Input: part model. Units: mm. Frame: model coordinates. Face numbers are marked on the shaded views. A direction names the side the tool comes from. Round coordinates to 2 decimals unless told otherwise and drop trailing zeros. Write each loop counter-clockwise with the first axis right and the second up, starting at its lowest first coordinate (ties: lowest second). Pieces come first, ordered by that corner, then holes. Notation, with made-up numbers: M -30,-30 L -5,-30 A25 ccw -5,-3 Z; hole C -3,68.5 d1. An arc over 180 degrees is marked long. Answer as CSV lines item,"result". Start each with the question number.
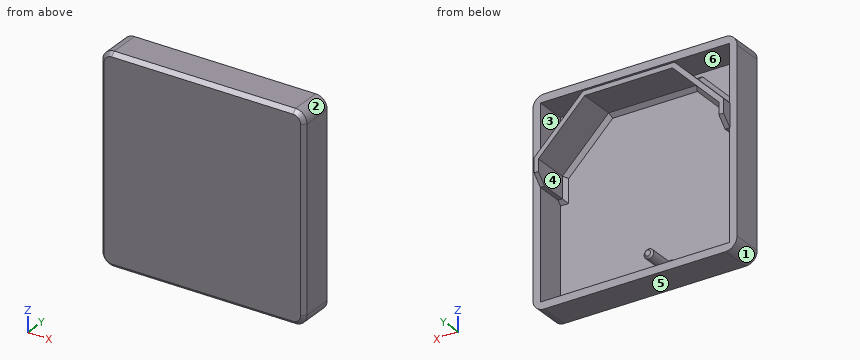
Autodesk Inventor part; units mm, degrees
ref_plane "YZ Plane" through (0, 0, 0) normal (1, 0, 0) x (0, 1, 0)
ref_plane "XZ Plane" through (0, 0, 0) normal (0, 1, 0) x (-1, 0, 0)
ref_plane "XY Plane" through (0, 0, 0) normal (0, 0, 1) x (1, 0, 0)
sketch "Náčrt1" plane through (0, 0, 0) normal (0, 1, 0) x (-1, 0, 0)
  line L0 (49.5, 49.5) -> (-49.5, 49.5)
  line L1 (-49.5, 49.5) -> (-49.5, -49.5)
  line L2 (-49.5, -49.5) -> (49.5, -49.5)
  line L3 (49.5, -49.5) -> (49.5, 49.5)
  line L4 (49.5, 49.5) -> (-49.5, -49.5) construction
  line L5 (-49.5, 49.5) -> (49.5, -49.5) construction
  line L6 (53.5, 53.5) -> (-53.5, 53.5)
  line L7 (-53.5, 53.5) -> (-53.5, -53.5)
  line L8 (-53.5, -53.5) -> (53.5, -53.5)
  line L9 (53.5, -53.5) -> (53.5, 53.5)
  line L10 (53.5, 53.5) -> (-53.5, -53.5) construction
  line L11 (-53.5, 53.5) -> (53.5, -53.5) construction
  point P0 (0, 0)
  dimension "d1" = 99
  dimension "d2" = 4
extrude "Vysunutí1" add sketch "Náčrt1" along normal blind 2 contours L3 L2 L1 L0
extrude "Vysunutí2" add sketch "Náčrt1" along normal blind 18
fillet "Zaoblení1" radius 6 4 edges at (53.5, 9, 53.5) (53.5, 9, -53.5) (-53.5, 9, -53.5) (-53.5, 9, 53.5)
chamfer "Zkosení1" distance 2 angle 45 8 edges at (0, 0, 53.5) (51.7426, 0, 51.7426) (53.5, 0, 0) (51.7426, 0, -51.7426) (0, 0, -53.5) (-51.7426, 0, -51.7426) (-53.5, 0, 0) (-51.7426, 0, 51.7426)
sketch "Náčrt2" plane through (0, 2, 0) normal (0, 1, 0) x (1, 0, 0)
  line L0 (47.25, -18.75) -> (23, -43)
  line L1 (23, -43) -> (-23, -43)
  line L2 (-23, -43) -> (-47.25, -18.75)
  line L3 (-49.75, -19.7855) -> (-24.0355, -45.5)
  line L4 (-24.0355, -45.5) -> (24.0355, -45.5)
  line L5 (24.0355, -45.5) -> (49.75, -19.7855)
  line L6 (49.75, -19.7855) -> (49.75, -7.5)
  line L7 (49.75, -7.5) -> (47.25, -7.5)
  line L8 (47.25, -7.5) -> (47.25, -18.75)
  line L9 (-47.25, -18.75) -> (-47.25, -7.5)
  line L10 (-47.25, -7.5) -> (-49.75, -7.5)
  line L11 (-49.75, -7.5) -> (-49.75, -19.7855)
  line L12 (49.5, -49.5) -> (-49.5, -49.5)
  line L13 (49.5, 49.5) -> (49.5, -49.5)
  point P0 (0, 0)
  point P1 (0, -45.5)
  point P2 (0, -49.5)
  point P3 (49.5, -20.0355)
  point P4 (49.5, -7.5)
  dimension "d12" = 2.5
  dimension "d13" = 2.5
  dimension "d14" = 2.5
  dimension "d15" = 46
  dimension "d16" = 135
  dimension "d17" = 2.5
  dimension "d18" = 2.5
  dimension "d19" = 38
  dimension "d20" = 99.5
  dimension "d21" = 11.25
  dimension "d22" = 4
extrude "Vysunutí3" add sketch "Náčrt2" along normal blind 21 contours L8 L7 L13 L5 L4 L3 L11 L10 L9 L2 L1 L0
sketch "Náčrt3" plane through (0, 2, 0) normal (0, 1, 0) x (1, 0, 0)
  circle A0 centre (-8, 43.25) radius 2.5
  circle A1 centre (-8, 43.25) radius 1.5
  line L0 (49.5, 49.5) -> (49.5, -7.5)
  line L1 (-49.5, -7.5) -> (-49.5, 49.5)
  line L2 (-49.5, 49.5) -> (49.5, 49.5)
  point P0 (0, 0)
  dimension "d27" = 3
  dimension "d28" = 5
  dimension "d39" = 41.5
  dimension "d43" = 6.25
extrude "Vysunutí4" add sketch "Náčrt3" along normal blind 18 contours A1
extrude "Vysunutí5" add sketch "Náčrt3" along normal blind 17
chamfer "Zkosení2" distance 1 angle 45 1 edges at (-9.5, 19, -43.25)
chamfer "Zkosení3" distance 2 angle 45 11 edges at (-10.5, 2, -43.25) (-35.125, 2, 30.875) (-47.25, 2, 13.125) (0, 2, 43) (35.125, 2, 30.875) (47.25, 2, 13.125) (48.375, 2, 7.5) (-48.375, 2, 7.5) (36.7678, 2, 32.7678) (0, 2, 45.5) (-36.7678, 2, 32.7678)
chamfer "Zkosení4" distance 5 angle 45 2 edges at (-48.5, 23, 7.5) (48.375, 23, 7.5)
properties part number "horni_vlozka"
Item 1: Cut plane A-A, the plane y = 10.5. Return loops of the section in (x, z).
Item 2: Line query: line 1 (Z direction, x = -14, y = 13.75); line 2 (X direction, y = 17, z = -4.5); line 3 (Z direction, x = 35.5, y = 17.25). Output: solid intervals per line, ascending. Write a range as [from, to].
Item 3: Access query for the marked faces 5 and 6. Directions: +Z, -Z, +X, -X, +Y, -Y. A direction counts if a zero-diameter tool reaches every point of the face in a straight line with its end or side. Return the directions, or none.
Item 4: Draft query along Z for the marked faces 1, 2, 3 and 4. Return one class per face: +Z half, -Z half, draft (parallel to the pull), parting line (faces both ways), or undercut.
Item 5: Pin query (flat end, axial travel): pin 1 Ø13.5 at (x, z) = (-17.5, 33) entering from +Y; pin 2 Ø0.7 at (x, y) = (48.5, 12.5) entering from -Z; pin 3 Ø5.5 at (x, z) = (-8, -44.5) entering from +Y. Return the tip coordinate at first contact, or that it passes through.
Item 6: Cut plane B-B, the plane z = -20.5. Return loops of the section in (x, y).
Results list:
1,outline,"M -53.5,-47.5 A6 ccw -47.5,-53.5 L 47.5,-53.5 A6 ccw 53.5,-47.5 L 53.5,47.5 A6 ccw 47.5,53.5 L -47.5,53.5 A6 ccw -53.5,47.5 Z; C -8,-43.25 d5; hole M -49.5,-49.5 L 49.5,-49.5 L 49.5,7.5 L 47.25,7.5 L 47.25,18.75 L 23,43 L -23,43 L -47.25,18.75 L -47.25,7.5 L -49.5,7.5 Z; hole M -49.5,20.04 L -24.04,45.5 L 24.04,45.5 L 49.5,20.04 L 49.5,49.5 L -49.5,49.5 Z"
2,line 1,"[-53.5, -49.5], [43, 45.5], [49.5, 53.5]"
2,line 2,"[-53.5, -49.5], [49.5, 53.5]"
2,line 3,"[-53.5, -49.5], [30.5, 34.04], [49.5, 53.5]"
3,face 5,"-Z, +X, -X, +Y, -Y"
3,face 6,"+Y"
4,face 1,"-Z half"
4,face 2,"+Z half"
4,face 3,"undercut"
4,face 4,"undercut"
5,pin 1,"y = 2"
5,pin 2,"z = -53.46"
5,pin 3,"y = 20"
6,outline,"M -53.5,2 L -51.5,0 L 51.5,0 L 53.5,2 L 53.5,18 L 49.5,18 L 49.5,2 L -49.5,2 L -49.5,18 L -53.5,18 Z"
